Could you check a few things on this model? Use its own coordinates, in mm. A direction names the side the tool comes from. Give positions to 0.01 mm unless a question says otherwise; leave off trailing zeros. Write each loop counter-clockwise with the first axis right and the second up, starting at its lowest first coordinate (ties: lowest second). Pieces come first, ordered by that corner, then holes. Notation, with made-up numbers: (78, 85) - (134, 85) arc R19 ccw to (134, 103) - close; hole circle Ø2 at (-32.75, 16.25). An arc over 180 degrees is marked (long way). Answer in a Markdown table with one row per item.
Autodesk Inventor part; units mm, degrees
ref_plane "YZ Plane" through (0, 0, 0) normal (1, 0, 0) x (0, 1, 0)
ref_plane "XZ Plane" through (0, 0, 0) normal (0, 1, 0) x (-1, 0, 0)
ref_plane "XY Plane" through (0, 0, 0) normal (0, 0, 1) x (1, 0, 0)
sketch "Sketch1" plane through (0, 0, 0) normal (0, 1, 0) x (-1, 0, 0)
  circle A0 centre (0, 0) radius 2.2
  dimension "d0" = 4.4
extrude "Extrusion1" add sketch "Sketch1" along normal blind 1
sketch "Sketch2" plane through (0, 1, 0) normal (0, 1, 0) x (1, 0, 0)
  line L0 (5, -6.6) -> (-5, -6.6)
  line L1 (-5, -6.6) -> (-5, 2.2)
  line L2 (-5, 2.2) -> (5, 2.2)
  line L3 (5, 2.2) -> (5, -6.6)
  circle A0 centre (0, 0) radius 2.2
  line L4 (5, -6.6) -> (-5, 2.2) construction
  line L5 (-5, -6.6) -> (5, 2.2) construction
  point P0 (0, -2.2)
  dimension "d3" = 10
extrude "Extrusion2" add sketch "Sketch2" along normal blind 0.7 contours A0 | L0 L1 L2 L3
sketch "Sketch3" plane through (0, 1.7, 0) normal (0, 1, 0) x (1, 0, 0)
  line L0 (-5, -6.6) -> (5, -6.6)
  line L1 (5, 2.2) -> (-5, 2.2)
  line L2 (-5, -6.6) -> (-4.3, -6.6)
  line L3 (-4.3, -6.6) -> (-4.3, 2.2)
  line L4 (-4.3, 2.2) -> (-5, 2.2)
  line L5 (-5, 2.2) -> (-5, -6.6)
  line L6 (5, 2.2) -> (4.3, 2.2)
  line L7 (4.3, 2.2) -> (4.3, -6.6)
  line L8 (4.3, -6.6) -> (5, -6.6)
  line L9 (5, -6.6) -> (5, 2.2)
  point P0 (0, 0)
  dimension "d6" = 0.7
  dimension "d7" = 0.7
extrude "Extrusion3" add sketch "Sketch3" along normal blind 8 contours L5 L1 L3 L0 | L7 L1 L9 L0
chamfer "Chamfer1" distance 0.3 angle 45 8 edges at (-5, 9.7, 2.2) (-5, 5.35, -2.2) (-5, 5.35, 6.6) (5, 9.7, 2.2) (5, 5.35, -2.2) (5, 5.35, 6.6) (5, 1, 2.2) (-5, 1, 2.2)
sketch "Sketch7" plane through (-5, 1.3, 6.3) normal (-1, 0, 0) x (0, 0, 1)
  line L0 (0, 0) -> (0, 8.1)
  line L1 (-8.2, 0) -> (0, 0)
  line L2 (0, 8.1) -> (-8.2, 0)
  line L3 (-8.2, 8.1) -> (-8.2, 0)
  line L4 (-4.1, 4.05) -> (-8.2, 4.05)
  line L5 (-8.2, 4.05) -> (-8.2, 8.1)
  line L6 (-8.2, 8.1) -> (-4.1, 8.1)
  line L7 (-4.1, 8.1) -> (-4.1, 4.05)
  line L8 (-4.1, 4.05) -> (-8.2, 4.05)
  line L9 (-8.2, 4.05) -> (-8.2, 7.55)
  line L10 (-8.2, 7.55) -> (-4.1, 7.55)
  line L11 (-4.1, 7.55) -> (-4.1, 4.05)
  circle A0 centre (-5.8287, 5.8) radius 0.75
  point P0 (-6.3, -1.3)
  dimension "d22" = 4.1
  dimension "d23" = 3.5
  dimension "d24" = 1.5
sketch "Sketch8" plane through (-5, 1.3, 6.3) normal (-1, 0, 0) x (0, 0, 1)
  point P0 (-6.3, -1.3)
extrude "Extrusion6" add sketch "Sketch7" along normal blind 3.8 contours A0
sketch "Sketch9" plane through (5, 1.3, -1.9) normal (1, 0, 0) x (0, 0, -1)
  circle A0 centre (-2.3713, 5.8) radius 0.75
  circle A1 centre (-2.3713, 5.8) radius 0.75
  point P0 (-1.9, -1.3)
extrude "Extrusion7" add sketch "Sketch9" along normal blind 3.8
properties part number "McCrea_arm-connector_Walle"
1) Will these pins go through, and if not, where does the flat tip stop? P1, Ø2.5, axis at x = 2, z = 4, coming from the -Y side; P2, Ø2, axis at y = 3, z = 3, coming from the +X side.
Check values:
| item | result |
|---|---|
| P1 | stops at y = 1 |
| P2 | stops at x = 5 |
2) On a 3-axis mill with a long thin cutter (end or side, diameter ignored), from which of +Z, -Z, +X, -X, +Y, -Y can I reach the whole of each face in a straight line? I mean faces 1 (the face through (8.8, 7, 0)), 2 (the face through (6.873, 7.832, 0.634)), 3 (the face through (-2.1, 0.49, -0.66)), 4 (the face through (-6.873, 7.832, 0.309)), 5 (the face through (4.3, 6, 2)). Say none if no direction works.
Check values:
| item | result |
|---|---|
| face 1 | +Z, -Z, +X, +Y, -Y |
| face 2 | +X |
| face 3 | -Y |
| face 4 | -X |
| face 5 | +Z, -Z, +Y |
3) Imagine slicing it at D-D (x = 1). List the corners of the cut face in (y, z) for me, then the cut area to 3 significant figures.
Check values:
| item | result |
|---|---|
| outline | (0, -1.96) - (1, -1.96) - (1, -2.2) - (1.7, -2.2) - (1.7, 6.6) - (1, 6.6) - (1, 1.96) - (0, 1.96) - close |
| area | 10.1 mm2 |
4) If I drill on line 1 (X direction, y = 9.25, z = -1); line 2 (X direction, y = 7.5, z = 1); line 3 (Y direction, x = -3.25, z = 1), over which ranges is the centre line in solid material (lowest first)?
Check values:
| item | result |
|---|---|
| line 1 | x = -5 to -4.3, 4.3 to 5 |
| line 2 | x = -8.8 to -4.3, 4.3 to 8.8 |
| line 3 | y = 1 to 1.7 |
5) Imagine slicing it at B-B (z = 0). List the corners of the cut face in (x, y) for me, then the cut area to 3 significant figures.
Check values:
| item | result |
|---|---|
| outline | (-8.8, 6.52) - (-5, 6.52) - (-5, 1.3) - (-4.7, 1) - (-2.2, 1) - (-2.2, 0) - (2.2, 0) - (2.2, 1) - (4.7, 1) - (5, 1.3) - (5, 6.52) - (8.8, 6.52) - (8.8, 7.68) - (5, 7.68) - (5, 9.4) - (4.7, 9.7) - (4.3, 9.7) - (4.3, 1.7) - (-4.3, 1.7) - (-4.3, 9.7) - (-4.7, 9.7) - (-5, 9.4) - (-5, 7.68) - (-8.8, 7.68) - close |
| area | 31.3 mm2 |
6) We'd pull the mould along X, two halves only. Please class faces 6 (the face through (0, 1.7, 2)), 7 (the face through (5, 5, 2)), 8 (the face through (0.4, 1.5, 6.6)): +X half, -X half, draft (parallel to the pull), parting line (faces both ways), or undercut.
Check values:
| item | result |
|---|---|
| face 6 | undercut |
| face 7 | +X half |
| face 8 | draft |
7) Imagine slicing it at A-A (y = 9). List the corners of the cut face in (x, z) for me.
Check values:
| item | result |
|---|---|
| outline | (-5, -1.9) - (-4.7, -2.2) - (-4.3, -2.2) - (-4.3, 6.6) - (-4.7, 6.6) - (-5, 6.3) - close; (4.3, -2.2) - (4.7, -2.2) - (5, -1.9) - (5, 6.3) - (4.7, 6.6) - (4.3, 6.6) - close |
8) Imagine slicing it at C-C (y = 7.1). List the corners of the cut face in (x, z) for me.
Check values:
| item | result |
|---|---|
| outline | (-8.8, -0.28) - (-5, -0.28) - (-5, -1.9) - (-4.7, -2.2) - (-4.3, -2.2) - (-4.3, 6.6) - (-4.7, 6.6) - (-5, 6.3) - (-5, 1.22) - (-8.8, 1.22) - close; (4.3, -2.2) - (4.7, -2.2) - (5, -1.9) - (5, -0.28) - (8.8, -0.28) - (8.8, 1.22) - (5, 1.22) - (5, 6.3) - (4.7, 6.6) - (4.3, 6.6) - close |
